from build123d import *

# Parameters (mm, degrees)
TABPAD_DEPTH               = 7
LIPPOCKETSKETCH001_W       = 3
LIPPOCKETSKETCH001_H       = 38.45
LIPGROOVEPOCKET_DEPTH      = 3
RAILHOLESSKETCH_R          = 2.3
RAILHOLESSKETCH_R_2        = 3.15
RAILHOLESPOCKET_DEPTH      = 7.001
OBJ1      = 1.6
OBJ2  = 7.001
TABCOUNTERBORESKETCH_R     = 3
TABCOUNTERBOREPOCKET_DEPTH = 3.5


with BuildPart() as part:
    # TabProfileSketch → TabPad (new body)
    with BuildSketch(Plane.XY):
        Polygon((-15, 0), (0, 0), (0, 3), (12, 3), (12, 41.45), (0, 41.45), (0, 44.45), (-15, 44.45), align=None)
    extrude(amount=-TABPAD_DEPTH)

    # LipPocketSketch001 → LipGroovePocket (cut)
    with BuildSketch(Plane.XY):
        with Locations((1.5, 22.225)):
            Rectangle(LIPPOCKETSKETCH001_W, LIPPOCKETSKETCH001_H)
    extrude(amount=-LIPGROOVEPOCKET_DEPTH, mode=Mode.SUBTRACT)

    # RailHolesSketch → RailHolesPocket (cut, through all)
    with BuildSketch(Plane.XY):
        with Locations((-7.5, 6.225)):
            Circle(RAILHOLESSKETCH_R)
        with Locations((-7.5, 22.225)):
            Circle(RAILHOLESSKETCH_R_2)
        with Locations((-7.5, 38.225)):
            Circle(RAILHOLESSKETCH_R)
    extrude(amount=-RAILHOLESPOCKET_DEPTH, mode=Mode.SUBTRACT)

    with BuildSketch(Plane.XY):
        with Locations((7, 11)):
            Circle(OBJ1)
        with Locations((7, 33.45)):
            Circle(OBJ1)
    extrude(amount=-OBJ2, mode=Mode.SUBTRACT)

    # TabCounterboreSketch → TabCounterborePocket (cut)
    with BuildSketch(Plane.XY):
        with Locations((7, 11)):
            Circle(TABCOUNTERBORESKETCH_R)
        with Locations((7, 33.45)):
            Circle(TABCOUNTERBORESKETCH_R)
    extrude(amount=-TABCOUNTERBOREPOCKET_DEPTH, mode=Mode.SUBTRACT)


solid = part.part
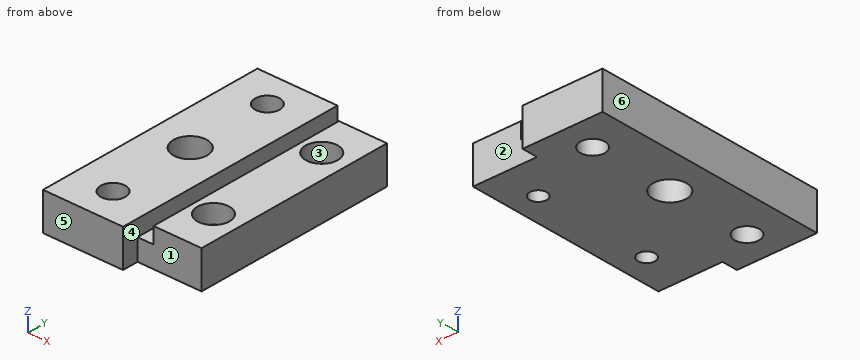
The model under review builds one solid part; all positions refer to its coordinate system, in mm. Face numbers are marked on the shaded views. A direction names the side the tool comes from. Round coordinates to 2 decimals unless told otherwise and drop trailing zeros. Loops run counter-clockwise (first coordinate to the right, second up) from the corner with the lowest first, then second, coordinate; pieces in that order, holes last. Notation, with made-up numbers: M 25,-26.5 L 76,-26.5 A26 cw 76,8.5 Z; hole C 70,-28.75 d5. An arc over 180 degrees is marked long. Answer as a JSON object with one key per item and string values.
Item 1: For line 1 along Y through (x, z) = (7, -2.55); line 2 along X through (y, z) = (22, -0.25); line 3 along X through (y, z) = (38, -2.75), list the stretches that pass through material, from the lowest coordinate up.
Check sheet entries:
{"line 1": "3 to 8, 14 to 30.45, 36.45 to 41.45", "line 2": "-15 to -10.64, -4.36 to 0, 3 to 12", "line 3": "-15 to -9.79, -5.21 to 0, 3 to 12"}
Item 2: We need section B-B, the plane y = 33.45. State the section outline as (x, z) points, and give its area (3 significant figures).
Check sheet entries:
{"outline": "M -15,-7 L 5.4,-7 L 5.4,-3.5 L 4,-3.5 L 4,0 L 3,0 L 3,-3 L 0,-3 L 0,0 L -15,0 Z; M 8.6,-7 L 12,-7 L 12,0 L 10,0 L 10,-3.5 L 8.6,-3.5 Z", "area": "148 mm2"}
Item 3: We need section A-A, the plane x = 7. State the section outline as (y, z) points.
Check sheet entries:
{"outline": "M 3,-7 L 9.4,-7 L 9.4,-3.5 L 8,-3.5 L 8,0 L 3,0 Z; M 12.6,-7 L 31.85,-7 L 31.85,-3.5 L 30.45,-3.5 L 30.45,0 L 14,0 L 14,-3.5 L 12.6,-3.5 Z; M 35.05,-7 L 41.45,-7 L 41.45,0 L 36.45,0 L 36.45,-3.5 L 35.05,-3.5 Z"}
Item 4: Clearance check with flat-ended pins moving along their axes: P1, Ø3.5, axis at x = 7, y = 11, coming from the +Z side; P2, Ø7.5, axis at x = -7.5, y = 6.225, coming from the +Z side; P3, Ø4, axis at x = -7.5, y = 22.225, coming from the -Z side; P4, Ø2, axis at x = 4.5, z = -2, coming from the +Y side. State where each tip first meets the part, or that it passes through.
Check sheet entries:
{"P1": "z = -3.5", "P2": "z = 0", "P3": "through", "P4": "y = 41.45"}
Item 5: The part is to be moulded in two halves that separate along X. For the marked faces 4, 5 and 6, say which applies: +X half, -X half, draft (parallel to the pull), parting line (faces both ways), or undercut.
Check sheet entries:
{"face 4": "undercut", "face 5": "draft", "face 6": "-X half"}
Item 6: We need section D-D, the plane z = -1. State the section outline as (x, y) points (3 decimals).
Check sheet entries:
{"outline": "M -15,0 L 0,0 L 0,44.45 L -15,44.45 Z; M 3,3 L 12,3 L 12,41.45 L 3,41.45 Z; hole C -7.5,22.225 d6.3; hole C -7.5,6.225 d4.6; hole C -7.5,38.225 d4.6; hole C 7,11 d6; hole C 7,33.45 d6"}
Item 7: We need section C-C, the plane x = -7.5. State the section outline as (y, z) points (3 decimals).
Check sheet entries:
{"outline": "M 0,-7 L 3.925,-7 L 3.925,0 L 0,0 Z; M 8.525,-7 L 19.075,-7 L 19.075,0 L 8.525,0 Z; M 25.375,-7 L 35.925,-7 L 35.925,0 L 25.375,0 Z; M 40.525,-7 L 44.45,-7 L 44.45,0 L 40.525,0 Z"}
Item 8: Tool access review of the marked faces 1, 2 and 3: name each direction out of +Z, -Z, +X, -X, +Y, -Y from which nothing blocks a thin tool from reaching the whole face with its end or side.
Check sheet entries:
{"face 1": "+Z, -Z, +X, -Y", "face 2": "+Z, -Z, +X, +Y", "face 3": "+Z"}
